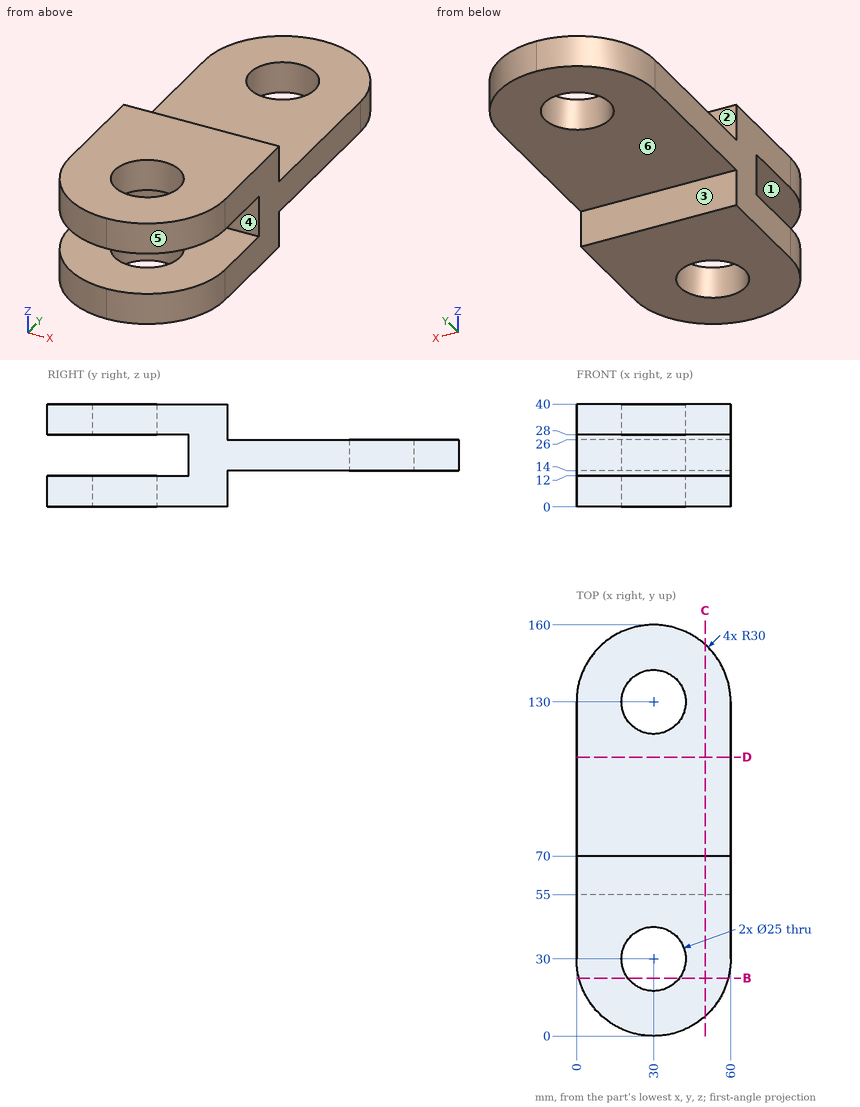
Verification items for this drawing (mm, ordinates from the low corner). A direction names the side the tool comes from. Give positions to 0.01 mm unless a question says otherwise; leave off trailing zeros. Write each loop counter-clockwise with the first axis right and the second up, starting at its lowest first coordinate (ties: lowest second). Pieces come first, ordered by that corner, then holes.
1) Set-up check for the marked faces 1, 2 and 3: record each of +Z, -Z, +X, -X, +Y, -Y from which the full face is reachable in a straight line by a thin tool's end or side.
Values follow:
face 1: +X, -X, -Y
face 2: +Z, +X, -X, +Y
face 3: -Z, +X, -X, +Y
2) Thickness scan on line 1 (Y direction, x = 30, z = 31); line 2 (Z direction, x = 16, y = 11); line 3 (X direction, y = 130, z = 17.75). Record the ranges inside material, lowest first.
Values follow:
line 1: y = 0 to 17.5, 42.5 to 70
line 2: z = 0 to 12, 28 to 40
line 3: x = 0 to 17.5, 42.5 to 60
3) Cross-section at D-D (y = 108.5). Record the boundary of the cut face in (x, z), plus the area to 3 significant figures.
Values follow:
outline: (0, 14) - (60, 14) - (60, 26) - (0, 26) - close
area: 720 mm2
4) Cross-section at C-C (x = 50). Record the boundary of the cut face in (y, z).
Values follow:
outline: (7.64, 0) - (70, 0) - (70, 14) - (152.36, 14) - (152.36, 26) - (70, 26) - (70, 40) - (7.64, 40) - (7.64, 28) - (55, 28) - (55, 12) - (7.64, 12) - close
5) Go/stop test with flat-tipped pins: pin 1 Ø8 at (y, z) = (138.5, 11.5) entering from +X; pin 2 Ø11 at (x, z) = (29, 5) entering from +Y; pin 3 Ø10 at (x, y) = (31, 117) entering from -Z. Record where each tip stops, or that it passes through.
Values follow:
pin 1: stops at x = 59.51
pin 2: stops at y = 70
pin 3: stops at z = 14
6) Release check for a two-part mould opening along Z. For the marked faces 4, 5 and 6 record: released by +Z, released by -Z, zero draft, split by the parting line, or undercut.
Values follow:
face 4: undercut
face 5: zero draft
face 6: released by -Z
7) Cross-section at B-B (y = 22.5). Record the boundary of the cut face in (x, z).
Values follow:
outline: (0.95, 0) - (20, 0) - (20, 12) - (0.95, 12) - close; (0.95, 28) - (20, 28) - (20, 40) - (0.95, 40) - close; (40, 0) - (59.05, 0) - (59.05, 12) - (40, 12) - close; (40, 28) - (59.05, 28) - (59.05, 40) - (40, 40) - close
